Answer from the drawing. Dimensions are ordinates in mm from the lowest x, y and z of the part. A direction names the side the tool comes from. Give positions to 0.01 mm unless a question says otherwise; leave off trailing zeros. Write each loop counter-clockwise with the first axis right and the second up, starting at its lowest first coordinate (ties: lowest second). Pieces come first, ordered by that corner, then holes. Notation, with made-up numbers: (44, 72) -> (86, 72) arc R35 ccw to (86, 111) -> close; hole circle Ø7 at (-33, 10). An arc over 180 degrees is marked (long way). Put each result on its own line as item: value. Start each with the question number.
1) Flat-ended cylindrical pins translate along their axes: pin 1 Ø2.5 at (x, y) = (4.5, 4.5) entering from -Z; pin 2 Ø3 at (y, z) = (4.5, 13) entering from +X; pin 3 Ø4 at (y, z) = (8.5, 14) entering from -X. Find the tip coordinate at first contact, or state that the pin passes through.
2) Find the intervals of material crossed by line 1 along Z through (x, y) = (6.5, 8); line 2 along Y through (x, z) = (5, 8.5); line 3 along Z through (x, y) = (3.75, 4.25), in increasing order. Write a range as from..to.
3) For a pull along Y with two mould halves and no side action, classify the marked faces 4, 5 and 6 as released by +Y, released by -Y, zero draft, split by the parting line, or undercut.
4) For the marked faces 1, 2 and 3, determine the directions among +Z, -Z, +X, -X, +Y, -Y from which every point of the face is accessible in a straight line to the end or side of a thin tool.
5) A cutting plane is placed at A-A (z = 10). Write down the section's boundary in (x, y), then the cut area to 3 significant figures.
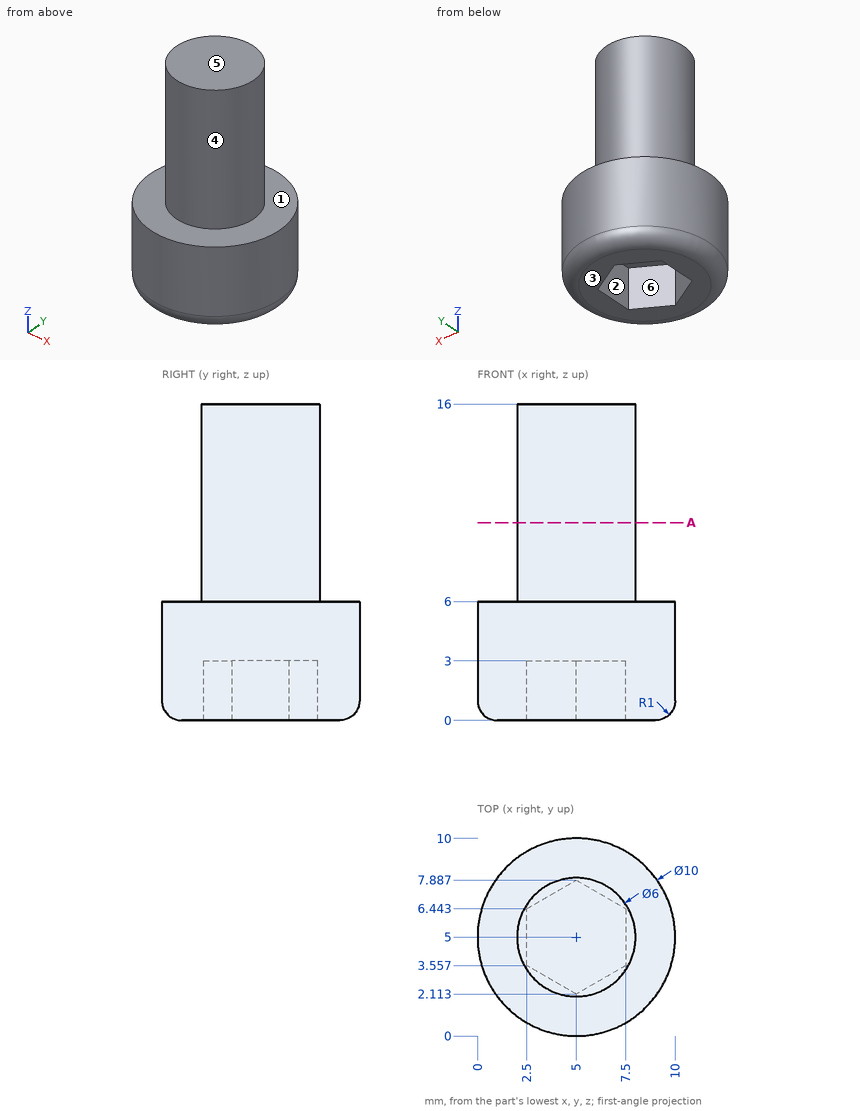
Reply:
1. pin 1: stops at z = 3
1. pin 2: stops at x = 8
1. pin 3: stops at x = 2.4
2. line 1: z = 0..6
2. line 2: y = 2..8
2. line 3: z = 3..16
3. face 4: split by the parting line
3. face 5: zero draft
3. face 6: undercut
4. face 1: +Z
4. face 2: -Z
4. face 3: -Z, +X, -X, +Y, -Y
5. outline: circle Ø6 at (5, 5)
5. area: 28.3 mm2
